Verification items for the finished model (mm, model axes). Face numbers are marked on the shaded views. A direction names the side the tool comes from. Give positions to 0.01 mm unless a question says otherwise; leave off trailing zeros. Write each loop counter-clockwise with the first axis right and the second up, starting at its lowest first coordinate (ties: lowest second). Pieces come first, ordered by that corner, then holes. Notation, with made-up numbers: (2.5, 26) -> (34.5, 26) arc R12 ccw to (34.5, 38) -> close; hole circle Ø4 at (81, 33). An arc over 180 degrees is marked (long way). Answer as CSV lines item,"result".
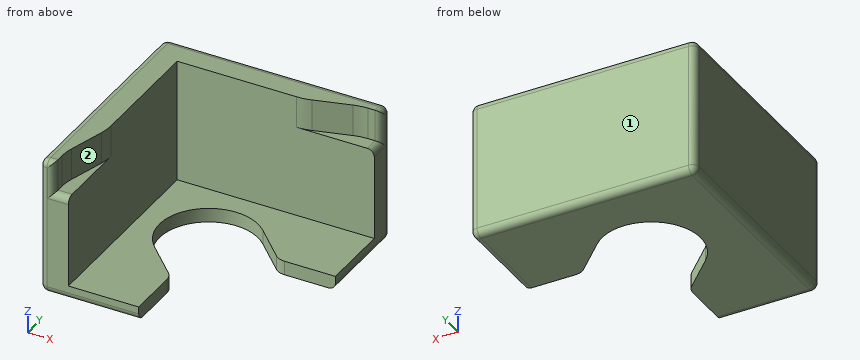
```python
from build123d import *

# Parameters (mm, degrees)
PAD_DEPTH    = 1
PAD001_DEPTH = 9.75
PAD002_DEPTH = 7.5
FILLET_R     = 0.49


with BuildPart() as part:
    # Sketch → Pad (new body)
    with BuildSketch(Plane.XY):
        with BuildLine():
            Line((0, 0), (0, -16))
            Line((0, -16), (7, -16))
            Line((7, -12.382704), (7, -16))
            ThreePointArc((7, -12.382704), (6.920435, -11.982704), (6.693853, -11.643601))
            Line((4.525126, -9.474874), (6.693853, -11.643601))
            ThreePointArc((9.474875, -4.525127), (4.525127, -4.525126), (4.525126, -9.474874))
            Line((9.474875, -4.525127), (11.643599, -6.693853))
            ThreePointArc((11.643599, -6.693853), (11.982703, -6.920435), (12.382703, -7))
            Line((12.382703, -7), (16, -7))
            Line((16, 0), (16, -7))
            Line((0, 0), (16, 0))
        make_face()
    extrude(amount=PAD_DEPTH)

    # Sketch001 (on XY_Plane of Origin) → Pad001 (join)
    with BuildSketch(Plane.XY):
        with BuildLine():
            Line((0, 0), (16, 0))
            Line((16, 0), (16, -1))
            Line((16, -1), (15.009808, -1))
            ThreePointArc((15.009808, -1), (14.504928, -1.035184), (14.009808, -1.140055))
            Line((14.009808, -1.140055), (11.490192, -1.859945))
            ThreePointArc((10.490192, -2), (10.995072, -1.964816), (11.490192, -1.859945))
            Line((10.490192, -2), (2, -2))
            Line((2, -2), (2, -10.490192))
            ThreePointArc((1.859945, -11.490192), (1.964816, -10.995072), (2, -10.490192))
            Line((1.859945, -11.490192), (1.140055, -14.009808))
            ThreePointArc((1.140055, -14.009808), (1.035184, -14.504928), (1, -15.009808))
            Line((1, -15.009808), (1, -16))
            Line((1, -16), (0, -16))
            Line((0, 0), (0, -16))
        make_face()
    extrude(amount=PAD001_DEPTH)

    # Sketch002 (on XY_Plane of Origin) → Pad002 (join)
    with BuildSketch(Plane.XY):
        Polygon((16, -2), (16, 0), (0, 0), (0, -16), (2, -16), (2, -2), align=None)
    extrude(amount=PAD002_DEPTH)

    # Fillet
    fillet_edges = [part.edges().sort_by_distance(p)[0] for p in [
        (1.5, -16, 7.5),
        (1, -16, 8.625),
        (0, -16, 4.875),
        (0.5, -16, 9.75),
        (0, -8, 9.75),
        (8, 0, 9.75),
        (16, -1, 8.625),
        (16, -0.5, 9.75),
        (16, 0, 4.875),
        (16, -1.5, 7.5),
        (0, 0, 4.875),
        (3.5, -16, 0),
        (16, -3.5, 0),
        (8, 0, 0),
        (0, -8, 0),
    ]]
    fillet(fillet_edges, radius=FILLET_R)


solid = part.part
```
1) Section check C-C (y = -13.25). Record the boundary of the cut face in (x, z).
Reported:
outline,"(0, 0.49) arc R0.49 ccw to (0.49, 0) -> (7, 0) -> (7, 1) -> (2, 1) -> (2, 7.5) -> (1.36, 7.5) -> (1.36, 9.75) -> (0.49, 9.75) arc R0.49 ccw to (0, 9.26) -> close"
2) Section check D-D (x = 14.5). Record the boundary of the cut face in (y, z).
Reported:
outline,"(-7, 0) -> (-0.49, 0) arc R0.49 ccw to (0, 0.49) -> (0, 9.26) arc R0.49 ccw to (-0.49, 9.75) -> (-1.04, 9.75) -> (-1.04, 7.5) -> (-2, 7.5) -> (-2, 1) -> (-7, 1) -> close"
3) Scan lines: line 1 along Y through (x, z) = (10.5, 9); line 2 along X through (y, z) = (-14.5, 6.25); line 3 along Z through (x, y) = (3.5, -10). Record each from-to range of solid material in increasing order.
Reported:
line 1,"-2 to 0"
line 2,"0 to 2"
line 3,"0 to 1"
4) Section check B-B (z = 6.25). Record the boundary of the cut face in (x, y), and give its area (3 significant figures).
Reported:
outline,"(0, -15.51) arc R0.49 ccw to (0.49, -16) -> (2, -16) -> (2, -2) -> (16, -2) -> (16, -0.49) arc R0.49 ccw to (15.51, 0) -> (0.49, 0) arc R0.49 ccw to (0, -0.49) -> close"
area,"59.8 mm²"
5) Section check A-A (x = 4.75). Record the boundary of the cut face in (y, z), and give its area (3 significant figures).
Reported:
outline,"(-16, 0.49) arc R0.49 ccw to (-15.51, 0) -> (-9.7, 0) -> (-9.7, 1) -> (-16, 1) -> close; (-4.32, 0) -> (-0.49, 0) arc R0.49 ccw to (0, 0.49) -> (0, 9.26) arc R0.49 ccw to (-0.49, 9.75) -> (-2, 9.75) -> (-2, 1) -> (-4.32, 1) -> close"
area,"28.0 mm²"
6) Tool access check on the marked faces 1 and 2. Record the directions out of +Z, -Z, +X, -X, +Y, -Y that give a thin tool (end or side, any length) a straight path to the whole face; none if there is none.
Reported:
face 1,"+Z, -Z, +X, -X, +Y"
face 2,"+Z, +X, -Y"
7) Depth check by flat-ended pin: pin 1 (4 mm diameter, centred on x = 12.5, y = -7, fed in from +Z); pin 2 (1.1 mm diameter, centred on x = 14.5, z = 0.5, fed in from -Y); pin 3 (0.5 mm diameter, centred on y = -13.5, z = 0.5, fed in from +X). Enter the tip coordinate at first touch or a pass-through.
Reported:
pin 1,"z = 1"
pin 2,"y = -7"
pin 3,"x = 7"
